```python
from build123d import *

# Parameters (mm, degrees)
F1_DEPTH       = 35
F3_D           = 5
F3_CSINK_D     = 10
F3_CSINK_ANGLE = 90
F6_D           = 5
F7_D           = 5
F9_D           = 5
F9_CSINK_D     = 10
F9_CSINK_ANGLE = 90


with BuildPart() as f1:
    # F0 (on Top) → F1 (new body)
    with BuildSketch(Plane.XY):
        Polygon((40, 40), (0, 0), (148.994949, 0), (108.994949, 40), align=None)
    extrude(amount=F1_DEPTH)

    # F3 (through all)
    with Locations(Plane.XZ):
        with Locations((74.497449, 17.5)):
            CounterSinkHole(F3_D / 2, F3_CSINK_D / 2, counter_sink_angle=F3_CSINK_ANGLE)

    # F6 (through all)
    with Locations(Plane(origin=(0, 0, 0), x_dir=(-0.707107, -0.707107, 0), z_dir=(-0.707107, 0.707107, 0))):
        with Locations((-28.284271, 17.5)):
            Hole(F6_D / 2)

    # F7 (through all)
    with Locations(Plane(origin=(74.497475, 74.497475, 0), x_dir=(-0.707107, 0.707107, 0), z_dir=(0.707107, 0.707107, 0))):
        with Locations((-77.071068, 17.5)):
            Hole(F7_D / 2)

    # F9 (through all)
    with Locations(Plane(origin=(0, 0, 0), x_dir=(1, 0, 0), z_dir=(0, 0, -1))):
        with Locations((102.781746, -25), (46.213203, -25)):
            CounterSinkHole(F9_D / 2, F9_CSINK_D / 2, counter_sink_angle=F9_CSINK_ANGLE)


solid = f1.part
```
Source: CAD feature listing. Evaluate the final solid. Frame: model axes, mm. Give positions to 0.01 mm unless a question says otherwise; leave off trailing zeros. Loops run counter-clockwise (first coordinate to the right, second up) from the corner with the lowest first, then second, coordinate; pieces in that order, holes last. Notation, with made-up numbers: (26.5, 31) -> (85.5, 31) arc R13 cw to (85.5, 56) -> close; hole circle Ø5 at (38, 81). An arc over 180 degrees is marked (long way). Use a Markdown table: item, result. Add a question column.
(1) Section query D-D (y = 14.5). Count the separate pieces of the cut face and the enclosed holes in it, then the cut area to 3 significant figures.
(2) Pull-direction query (Z, two-part tool) for faces 1 (the face through (129.275, 19.72, 21.144)), 2 (the face through (116.156, 10.693, 17.61)), 3 (the face through (105.4, 24.88, 2.38)); classes: +Z half, -Z half, draft (parallel to the pull), parting line (faces both ways), or undercut.
(3) Section query C-C (z = 26.5). Output: boundary loops of the cut face in (x, y), then the cut area to 3 significant figures.
(4) Ray query, line 1 (X direction, y = 25, z = 28); line 2 (X direction, y = 24, z = 4); line 3 (X direction, y = 11, z = 17). Return the intervals inside material, ascending.
(5) Section query A-A (z = 17.5). Output: boundary loops of the cut face in (x, y).
(6) Section query B-B (y = 25). Output: boundary loops of the cut face in (x, z).
(7) First-contact query: pin 1 Ø4 at (x, y) = (46.21, 25) entering from +Z; pin 2 Ø4 at (y, z) = (34, 4.5) entering from -X; pin 3 Ø6 at (y, z) = (31.5, 7.5) entering from +X; pin 4 Ø12 at (y, z) = (9, 24) entering from +X. Flat tips, straight axial feed; report the tip coordinate or a pass-through.
Checked values:
| question | item | result |
|---|---|---|
| 1 | separate pieces | 1 |
| 1 | enclosed holes | 3 |
| 1 | area | 4,120 mm^2 |
| 2 | face 1 | draft |
| 2 | face 2 | undercut |
| 2 | face 3 | -Z half |
| 3 | outline | (0, 0) -> (148.99, 0) -> (108.99, 40) -> (40, 40) -> close; hole circle Ø5 at (46.21, 25); hole circle Ø5 at (102.78, 25) |
| 3 | area | 4,320 mm^2 |
| 4 | line 1 | 25 to 43.71, 48.71 to 100.28, 105.28 to 123.99 |
| 4 | line 2 | 24 to 43.92, 48.5 to 100.49, 105.07 to 124.99 |
| 4 | line 3 | 11 to 25.54, 32.46 to 72.05, 76.95 to 116.53, 123.46 to 137.99 |
| 5 | outline | (0, 0) -> (36.46, 0) -> (18.23, 18.23) -> close; (21.77, 21.77) -> (43.54, 0) -> (69.5, 0) -> (72, 2.5) -> (72, 40) -> (40, 40) -> close; (77, 2.5) -> (79.5, 0) -> (105.46, 0) -> (127.23, 21.77) -> (108.99, 40) -> (77, 40) -> close; (112.53, 0) -> (148.99, 0) -> (130.76, 18.23) -> close; hole circle Ø5 at (46.21, 25); hole circle Ø5 at (102.78, 25) |
| 6 | outline | (25, 0) -> (41.21, 0) -> (43.71, 2.5) -> (43.71, 35) -> (25, 35) -> close; (48.71, 2.5) -> (51.21, 0) -> (97.78, 0) -> (100.28, 2.5) -> (100.28, 35) -> (48.71, 35) -> close; (105.28, 2.5) -> (107.78, 0) -> (123.99, 0) -> (123.99, 35) -> (105.28, 35) -> close; hole circle Ø5 at (74.5, 17.5) |
| 7 | pin 1 | through |
| 7 | pin 2 | x = 32 |
| 7 | pin 3 | x = 120.49 |
| 7 | pin 4 | x = 145.99 |
